Source: CAD feature listing. Evaluate the final solid. Frame: model axes, mm. A direction names the side the tool comes from. Round coordinates to 2 decimals unless told otherwise and drop trailing zeros. Write each loop counter-clockwise with the first axis right and the second up, starting at its lowest first coordinate (ties: lowest second). Pieces come first, ordered by that corner, then holes.
from build123d import *

# Parameters (mm, degrees)
SKETCH_3_R             = 5.5
EXTRUDE_2_DEPTH        = 4
SKETCH_4_R             = 4.25
EXTRUDE_3_DEPTH        = 20
CUT_EXTRUDE_1_DEPTH    = 10
HOLE_WIZARD_M5_1_D     = 4.2
HOLE_WIZARD_M5_1_DEPTH = 12.4
HOLE_WIZARD_M5_1_TIP   = 1.2618073


with BuildPart() as part:
    # Sketch 1 → Revolve 1 (revolve)
    with BuildSketch(Plane.XY):
        with BuildLine():
            Line((-4, 3.854610875), (-4, 2.495599217))
            Line((-4, 2.495599217), (4, 2.504403811))
            Line((4, 2.504403811), (4, 3.854610875))
            ThreePointArc((4, 3.854610875), (3.523970046, 4.294142536), (3, 4.675256677))
            Line((3, 4.675256677), (3, 8.485281374))
            ThreePointArc((3, 8.485281374), (0, 9), (-3, 8.485281374))
            Line((-3, 8.485281374), (-3, 4.675256677))
            ThreePointArc((-3, 4.675256677), (-3.523970046, 4.294142536), (-4, 3.854610875))
        make_face()
    revolve(axis=Axis((3.999995155, 0.004402291, 0), (-0.999999394, -0.001100574, 0)))



with BuildPart() as body_2:
    # Sketch 3 → Extrude 2 (new body)
    with BuildSketch(Plane.XY.offset(27)):
        Circle(SKETCH_3_R)
    extrude(amount=EXTRUDE_2_DEPTH)


with BuildPart() as part_1:
    add(part.part)

    add(body_2.part)  # Extrude 3 merges body 2
    # Sketch 4 → Extrude 3 (add)
    with BuildSketch(Plane(origin=(0, 0, 27), x_dir=(-1, 0, 0), z_dir=(0, 0, -1))):
        Circle(SKETCH_4_R)
    extrude(amount=EXTRUDE_3_DEPTH)

    # Sketch 5 → Cut-Extrude 1 (cut, symmetric)
    with BuildSketch(Plane(origin=(0, 0, 0), x_dir=(1, 0, 0), z_dir=(0, 1, 0))):
        Polygon((-2.994932477, -7), (-2.994932477, -7.933315826), (-4.25, -10), (-4.25, -7), align=None)
        Polygon((4.25, -7), (2.994932477, -7), (2.994932477, -7.933315826), (4.25, -10), align=None)
    extrude(amount=CUT_EXTRUDE_1_DEPTH, both=True, mode=Mode.SUBTRACT)

    # Hole Wizard M5 _1
    with Locations(Plane.XY.offset(31)):
        with Locations((0, 0)):
            Hole(HOLE_WIZARD_M5_1_D / 2, depth=HOLE_WIZARD_M5_1_DEPTH)
            with Locations((0, 0, -(HOLE_WIZARD_M5_1_DEPTH + HOLE_WIZARD_M5_1_TIP / 2))):  # 118° drill point
                Cone(0, HOLE_WIZARD_M5_1_D / 2, HOLE_WIZARD_M5_1_TIP, mode=Mode.SUBTRACT)


solid = part_1.part
1) Section query A-A on z = 14.5. Return the cut outline in (x, y).
Taken from the geometry:
outline: circle Ø8.5 at (0, 0)
2) Contact query for flat-ended pins moving along their axis: P1, Ø3, axis at y = 1, z = 16.5, coming from the +X side; P2, Ø8, axis at y = 1, z = -2.5, coming from the +X side; P3, Ø1.5, axis at x = 1.5, y = 2.5, coming from the -Z side. Output: stop coordinate, or through.
Taken from the geometry:
P1: stops at x = 4.25
P2: stops at x = 4.01
P3: stops at z = -8.74
3) Reachability of faces 5 (the face through (0.553, 4.214, 17.14)), 6 (the face through (2.995, 0.1, 7.5)), 7 (the face through (-2.994, -0.636, -4.822)) from +Z, -Z, +X, -X, +Y, -Y: full face, straight path, thin tool, end or side. Return the list, or none.
Taken from the geometry:
face 5: none
face 6: +X, +Y, -Y
face 7: -X
4) Material intervals for line 1 (X direction, y = 0, z = 22.5); line 2 (Z direction, x = 4.25, y = -2.75), sorted ascending.
Taken from the geometry:
line 1: x = -4.25 to -2.1, 2.1 to 4.25
line 2: z = 27 to 31
5) Pull-direction query (Y, two-part tool) for faces 1 (the face through (-1.19, -5.37, 28.97)), 2 (the face through (0.35, 0.11, 17.56)), 3 (the face through (0.06, -0.33, -2.48)), 4 (the face through (-0.1, -2.4, 31)); classes: released by +Y, released by -Y, zero draft, split by the parting line, or undercut.
Taken from the geometry:
face 1: split by the parting line
face 2: undercut
face 3: undercut
face 4: zero draft
